The figure shows three views and two pictorial views of one solid part (mm, origin at its lowest corner). Answer the questions. A direction names the side the tool comes from. Round coordinates to 2 decimals unless told otherwise and drop trailing zeros. Write each loop counter-clockwise with the first axis right and the second up, starting at its lowest first coordinate (ties: lowest second). Pieces come first, ordered by that corner, then holes.
Item 1: Find section A-A on y = 12.5. Give the vertices of the cut face in (x, z).
Item 2: Find section B-B on x = 18.9. Give the vertices of the cut face in (y, z), then the cut area to 3 significant figures.
Item 3: For a pull along X with two mould halves and no side action, classify the marked faces 5, 6, 7 and 8 as +X half, -X half, draft (parallel to the pull), parting line (faces both ways), or undercut.
Item 4: Find section C-C on z = 14. Give the vertices of the cut face in (x, y), then the cut area to 3 significant figures.
Item 5: Each of these flat-tipped pins is pushed along its axis until it touches: pin 1 (7.5 mm diameter, centred on x = 6.9, z = 14, fed in from -Y); pin 2 (1.7 mm diameter, centred on y = 2, z = 5.5, fed in from +X); pin 3 (2.5 mm diameter, centred on x = 18.9, z = 14, fed in from -Y); pin 4 (3 mm diameter, centred on y = 4, z = 3, fed in from -X). Where does it stop, or does it pass through?
Item 6: A tool of negligible diameter and unlimited length cuts with its end or side. For the marked faces 1, 2, 3 and 4, from which of +Z, -Z, +X, -X, +Y, -Y can it reach the whole face along a straight path? Write none if from no direction.
Item 7: Find section D-D on z = 5.5. Give the vertices of the cut face in (x, y).
Item 8: Find the intervals of material crossed by probe 1 along Z at (x, y) = (18.9, 16.25); probe 2 along Z at (x, y) = (18.9, 12); probe 3 along X at (y, z) = (19.25, 14.75), in increasing order.
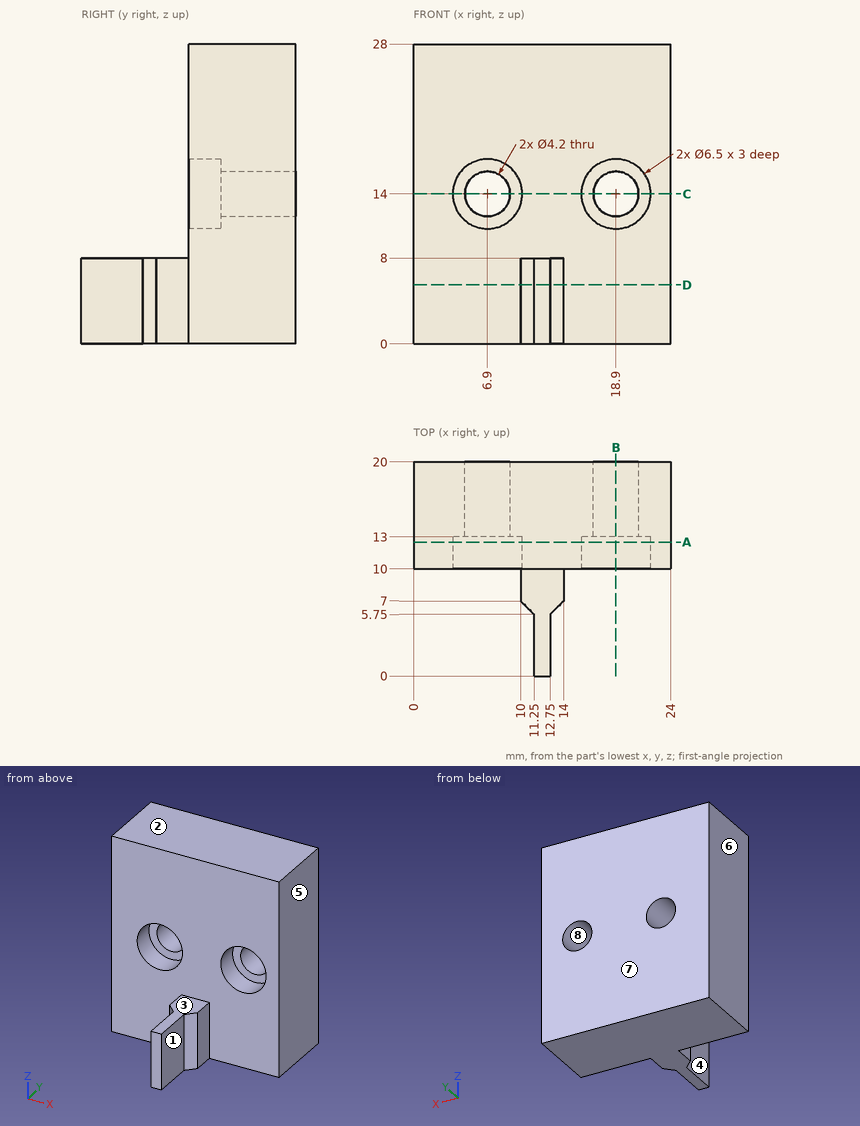
Check values:
1. outline: (0, 0) - (24, 0) - (24, 28) - (0, 28) - close; hole circle Ø6.5 at (6.9, 14); hole circle Ø6.5 at (18.9, 14)
2. outline: (10, 0) - (20, 0) - (20, 11.9) - (13, 11.9) - (13, 10.75) - (10, 10.75) - close; (10, 17.25) - (13, 17.25) - (13, 16.1) - (20, 16.1) - (20, 28) - (10, 28) - close
2. area: 231 mm2
3. face 5: +X half
3. face 6: -X half
3. face 7: draft
3. face 8: undercut
4. outline: (0, 10) - (3.65, 10) - (3.65, 13) - (4.8, 13) - (4.8, 20) - (0, 20) - close; (9, 13) - (10.15, 13) - (10.15, 10) - (15.65, 10) - (15.65, 13) - (16.8, 13) - (16.8, 20) - (9, 20) - close; (21, 13) - (22.15, 13) - (22.15, 10) - (24, 10) - (24, 20) - (21, 20) - close
4. area: 142 mm2
5. pin 1: stops at y = 10
5. pin 2: stops at x = 12.75
5. pin 3: passes through
5. pin 4: stops at x = 11.25
6. face 1: +Z, -Z, +X, -Y
6. face 2: +Z, +X, -X, +Y, -Y
6. face 3: +Z, +X, -X, -Y
6. face 4: +Z, -Z, -X, -Y
7. outline: (0, 10) - (10, 10) - (10, 7) - (11.25, 5.75) - (11.25, 0) - (12.75, 0) - (12.75, 5.75) - (14, 7) - (14, 10) - (24, 10) - (24, 20) - (0, 20) - close
8. probe 1: z = 0 to 11.9, 16.1 to 28
8. probe 2: z = 0 to 10.75, 17.25 to 28
8. probe 3: x = 0 to 4.94, 8.86 to 16.94, 20.86 to 24
